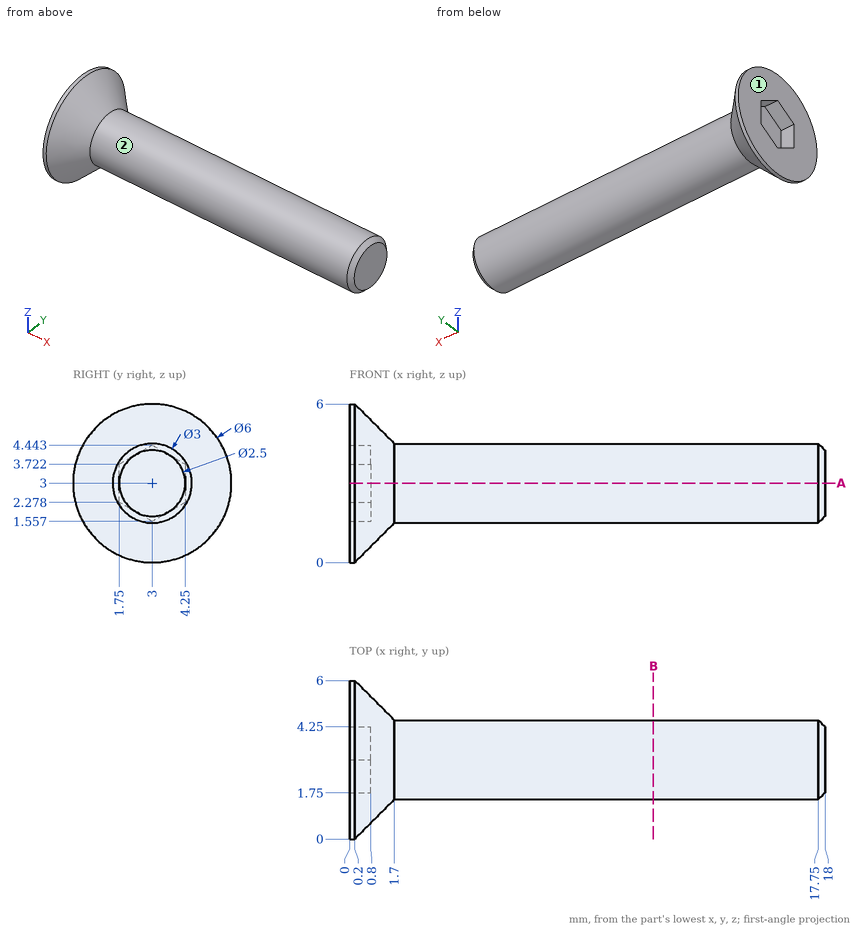
Geometry check sheet. Reference: drawing and pictorial views, mm from the part's lowest x, y, z. A direction names the side the tool comes from. Give positions to 0.01 mm unless a question says otherwise; leave off trailing zeros. Loops run counter-clockwise (first coordinate to the right, second up) from the corner with the lowest first, then second, coordinate; pieces in that order, holes last. Notation, with made-up numbers: (-37.75, -11.5) -> (-19.75, -11.5) arc R21 cw to (-19.75, -7.5) -> close; hole circle Ø1 at (-21, 12). An arc over 180 degrees is marked (long way). Answer in a Markdown table with one row per item. Add a question column.
1) Cross-section at B-B on x = 11.5. Record the boundary of the cut face in (y, z).
2) Material ranges on probe 1 along Z at (x, y) = (10.25, 3.4) (1 decimal); probe 2 along X at (y, z) = (2.6, 2.1); probe 3 along Y at (x, z) = (7.25, 3.9), recorded low to high. Write a range as from..to.
3) Cross-section at A-A on z = 3. Record the boundary of the cut face in (x, y).
4) Gauge pin test, flat ends, axial feed: P1, Ø3, axis at x = 7.5, z = 2.5, coming from the -Y side; P2, Ø1, axis at y = 1, z = 1.5, coming from the +X side; P3, Ø2, axis at x = 6, z = 5, coming from the +Y side. Record the tip position at first contact, or that the pin passes through.
5) Set-up check for the marked faces 1 and 2: record each of +Z, -Z, +X, -X, +Y, -Y from which the full face is reachable in a straight line by a thin tool's end or side.
Outcome:
| question | item | result |
|---|---|---|
| 1 | outline | circle Ø3 at (3, 3) |
| 2 | probe 1 | z = 1.6..4.4 |
| 2 | probe 2 | x = 0.8..18 |
| 2 | probe 3 | y = 1.8..4.2 |
| 3 | outline | (0, 0) -> (0.2, 0) -> (1.7, 1.5) -> (17.75, 1.5) -> (18, 1.75) -> (18, 4.25) -> (17.75, 4.5) -> (1.7, 4.5) -> (0.2, 6) -> (0, 6) -> (0, 4.25) -> (0.8, 4.25) -> (0.8, 1.75) -> (0, 1.75) -> close |
| 4 | P1 | stops at y = 1.5 |
| 4 | P2 | stops at x = 1.2 |
| 4 | P3 | stops at y = 4.12 |
| 5 | face 1 | +Z, -Z, -X, +Y, -Y |
| 5 | face 2 | +X |
